```python
from build123d import *

# Parameters (mm, degrees)
SKETCH2_R                           = 3.35
F_80_SERIES_TS80_80M_650039_2_DEPTH = 720
M8X1_25_TAPPED_HOLE2_D              = 6.8
M8X1_25_TAPPED_HOLE2_DEPTH          = 25
M8X1_25_TAPPED_HOLE2_TIP            = 2.042926105
M8X1_25_TAPPED_HOLE3_D              = 6.8
M8X1_25_TAPPED_HOLE3_DEPTH          = 25
M8X1_25_TAPPED_HOLE3_TIP            = 2.042926105


with BuildPart() as part:
    # Sketch2 → 80 series TS80-80M-650039(2) (new body)
    with BuildSketch(Plane(origin=(0, 0, 0), x_dir=(-1, 0, 0), z_dir=(0, 1, 0))):
        with BuildLine():
            Line((-28, 15.179010667), (-28, 24.820989333))
            Line((-28, 24.820989333), (-35.5438, 32.364789333))
            Line((-35.5438, 32.364789333), (-35.5438, 24))
            Line((-35.5438, 24), (-40, 24))
            Line((-40, 24), (-40, 37))
            ThreePointArc((-40, 37), (-39.121320344, 39.121320344), (-37, 40))
            Line((-37, 40), (-24, 40))
            Line((-24, 40), (-24, 35.301))
            Line((-24, 35.301), (-32.121989333, 35.301))
            Line((-32.121989333, 35.301), (-24.820989333, 28))
            Line((-24.820989333, 28), (-15.179010667, 28))
            Line((-15.179010667, 28), (-7.878010667, 35.301))
            Line((-7.878010667, 35.301), (-16, 35.301))
            Line((-16, 35.301), (-16, 40))
            Line((-16, 40), (16, 40))
            Line((16, 40), (16, 35.301))
            Line((16, 35.301), (7.878010667, 35.301))
            Line((7.878010667, 35.301), (15.179010667, 28))
            Line((15.179010667, 28), (24.820989333, 28))
            Line((24.820989333, 28), (32.121989333, 35.301))
            Line((32.121989333, 35.301), (24, 35.301))
            Line((24, 35.301), (24, 40))
            Line((24, 40), (37, 40))
            ThreePointArc((37, 40), (39.121320344, 39.121320344), (40, 37))
            Line((40, 37), (40, 24))
            Line((40, 24), (35.5438, 24))
            Line((35.5438, 24), (35.5438, 32.364789333))
            Line((35.5438, 32.364789333), (28, 24.820989333))
            Line((28, 24.820989333), (28, 15.179010667))
            Line((28, 15.179010667), (35.5438, 7.635210667))
            Line((35.5438, 7.635210667), (35.5438, 16))
            Line((35.5438, 16), (40, 16))
            Line((40, 16), (40, -16))
            Line((40, -16), (35.5438, -16))
            Line((35.5438, -16), (35.5438, -7.635210667))
            Line((35.5438, -7.635210667), (28, -15.179010667))
            Line((28, -15.179010667), (28, -24.820989333))
            Line((28, -24.820989333), (35.5438, -32.364789333))
            Line((35.5438, -32.364789333), (35.5438, -24))
            Line((35.5438, -24), (40, -24))
            Line((40, -24), (40, -37))
            ThreePointArc((40, -37), (39.121320344, -39.121320344), (37, -40))
            Line((37, -40), (24, -40))
            Line((24, -40), (24, -35.301))
            Line((24, -35.301), (32.121989333, -35.301))
            Line((32.121989333, -35.301), (24.820989333, -28))
            Line((24.820989333, -28), (15.179010667, -28))
            Line((15.179010667, -28), (7.878010667, -35.301))
            Line((7.878010667, -35.301), (16, -35.301))
            Line((16, -35.301), (16, -40))
            Line((16, -40), (-16, -40))
            Line((-16, -40), (-16, -35.301))
            Line((-16, -35.301), (-7.878010667, -35.301))
            Line((-7.878010667, -35.301), (-15.179010667, -28))
            Line((-15.179010667, -28), (-24.820989333, -28))
            Line((-24.820989333, -28), (-32.121989333, -35.301))
            Line((-32.121989333, -35.301), (-24, -35.301))
            Line((-24, -35.301), (-24, -40))
            Line((-24, -40), (-37, -40))
            ThreePointArc((-37, -40), (-39.121320344, -39.121320344), (-40, -37))
            Line((-40, -37), (-40, -24))
            Line((-40, -24), (-35.5438, -24))
            Line((-35.5438, -24), (-35.5438, -32.364789333))
            Line((-35.5438, -32.364789333), (-28, -24.820989333))
            Line((-28, -24.820989333), (-28, -15.179010667))
            Line((-28, -15.179010667), (-35.5438, -7.635210667))
            Line((-35.5438, -7.635210667), (-35.5438, -16))
            Line((-35.5438, -16), (-40, -16))
            Line((-40, -16), (-40, 16))
            Line((-40, 16), (-35.5438, 16))
            Line((-35.5438, 16), (-35.5438, 7.635210667))
            Line((-35.5438, 7.635210667), (-28, 15.179010667))
        make_face()
        with Locations((20, -20)):
            Circle(SKETCH2_R, mode=Mode.SUBTRACT)
        with Locations((-20, -20)):
            Circle(SKETCH2_R, mode=Mode.SUBTRACT)
        with Locations((-20, 20)):
            Circle(SKETCH2_R, mode=Mode.SUBTRACT)
        with Locations((20, 20)):
            Circle(SKETCH2_R, mode=Mode.SUBTRACT)
        Polygon((-11.353421559, 24.174410892), (0, 35.527832452), (11.353421559, 24.174410892), (11.353421559, 11.353421559), (24.174410892, 11.353421559), (35.527832452, 0), (24.174410892, -11.353421559), (11.353421559, -11.353421559), (11.353421559, -24.174410892), (0, -35.527832452), (-11.353421559, -24.174410892), (-11.353421559, -11.353421559), (-24.174410892, -11.353421559), (-35.527832452, 0), (-24.174410892, 11.353421559), (-11.353421559, 11.353421559), align=None, mode=Mode.SUBTRACT)
    extrude(amount=F_80_SERIES_TS80_80M_650039_2_DEPTH)

    # M8x1.25 Tapped Hole2
    with Locations(Plane(origin=(0, 0, 0), x_dir=(-1, 0, 0), z_dir=(0, -1, 0))):
        with Locations((-20, 20), (20, 20), (20, -20), (-20, -20)):
            Hole(M8X1_25_TAPPED_HOLE2_D / 2, depth=M8X1_25_TAPPED_HOLE2_DEPTH)
            with Locations((0, 0, -(M8X1_25_TAPPED_HOLE2_DEPTH + M8X1_25_TAPPED_HOLE2_TIP / 2))):  # 118° drill point
                Cone(0, M8X1_25_TAPPED_HOLE2_D / 2, M8X1_25_TAPPED_HOLE2_TIP, mode=Mode.SUBTRACT)

    # M8x1.25 Tapped Hole3
    with Locations(Plane(origin=(0, 720, 0), x_dir=(1, 0, 0), z_dir=(0, 1, 0))):
        with Locations((-20, -20)):
            Hole(M8X1_25_TAPPED_HOLE3_D / 2, depth=M8X1_25_TAPPED_HOLE3_DEPTH)
            with Locations((0, 0, -(M8X1_25_TAPPED_HOLE3_DEPTH + M8X1_25_TAPPED_HOLE3_TIP / 2))):  # 118° drill point
                Cone(0, M8X1_25_TAPPED_HOLE3_D / 2, M8X1_25_TAPPED_HOLE3_TIP, mode=Mode.SUBTRACT)


solid = part.part
```
Geometry: final body of the model. Coordinates: model frame, mm. A direction names the side the tool comes from. Round coordinates to 2 decimals unless told otherwise and drop trailing zeros. Use CSV: the item, a comma, the result in double quotes. Start each with the question number.
Q1. First-contact query: pin 1 Ø3 at (y, z) = (499.5, -19.5) entering from +X. Flat tip, straight axial feed; report the tip coordinate or a pass-through.
Q2. Reachability of faces 4 (the face through (0, 355, -40)), 5 (the face through (18, 355, 11.353)) from +Z, -Z, +X, -X, +Y, -Y: full face, straight path, thin tool, end or side. Return the list, or none.
Q3. Section A-A (y = 206). Give the number of separate pieces and of enclosed holes in the cut face, plus the area to 3 significant figures.
Q4. Line query: L1, parallel to X at y = 5, z = 20; L2, parallel to Z at x = 20, y = 322. Output: solid intervals per line, ascending.
Q5. Pull-direction query (X, two-part tool) for faces 1 (the face through (40, 355, 0)), 2 (the face through (-30, 355, 40)), 3 (the face through (-29.93, 354.96, -5.6)); classes: pulls with the +X half, pulls with the -X half, needs draft (parallel to the pull), parting line crosses it, or undercut.
Result sheet:
1,pin 1,"x = 28"
2,face 4,"-Z, +X, -X, +Y, -Y"
2,face 5,"+Y, -Y"
3,separate pieces,"1"
3,enclosed holes,"5"
3,area,"2,750 mm²"
4,L1,"-28 to -23.4, -16.6 to -11.35, 11.35 to 16.6, 23.4 to 28"
4,L2,"-28 to -23.35, -16.65 to -11.35, 11.35 to 16.65, 23.35 to 28"
5,face 1,"pulls with the +X half"
5,face 2,"needs draft"
5,face 3,"undercut"
